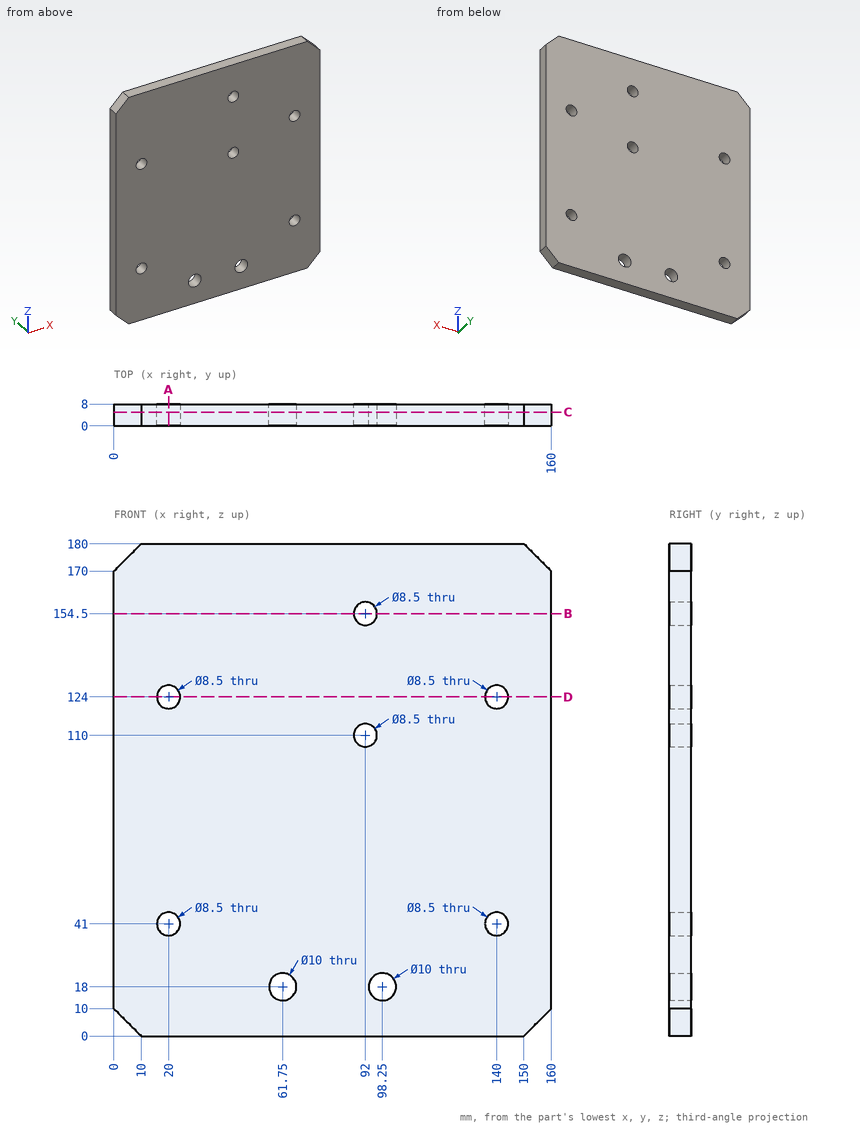
Geometry check sheet. Reference: drawing and pictorial views, mm from the part's lowest x, y, z. Give positions to 0.01 mm unless a question says otherwise; leave off trailing zeros. Order: outer loops, then holes, each group sorted by start corner. A loop starts at its lowest first (then second) coordinate and runs counter-clockwise, first axis right, second up.
1. Section check B-B, the plane z = 154.5. Enter the section's corners in (x, y).
2. Section check D-D, the plane z = 124. Enter the section's corners in (x, y).
3. Section check C-C, the plane y = 5. Give the number of separate pieces and of enclosed holes in the cut face, and give its area (3 significant figures).
4. Section check A-A, the plane x = 20. Enter the section's corners in (y, z).
5. Thickness scan on L1, parallel to Z at x = 92, y = 2; L2, parallel to Z at x = 140, y = 5.75; L3, parallel to Z at x = 61.75, y = 6.5. Record the ranges inside material, lowest first.
Values follow:
1. outline: (0, 0) - (87.75, 0) - (87.75, 8) - (0, 8) - close; (96.25, 0) - (160, 0) - (160, 8) - (96.25, 8) - close
2. outline: (0, 0) - (15.75, 0) - (15.75, 8) - (0, 8) - close; (24.25, 0) - (135.75, 0) - (135.75, 8) - (24.25, 8) - close; (144.25, 0) - (160, 0) - (160, 8) - (144.25, 8) - close
3. separate pieces: 1
3. enclosed holes: 8
3. area: 28,100 mm2
4. outline: (0, 0) - (8, 0) - (8, 36.75) - (0, 36.75) - close; (0, 45.25) - (8, 45.25) - (8, 119.75) - (0, 119.75) - close; (0, 128.25) - (8, 128.25) - (8, 180) - (0, 180) - close
5. L1: z = 0 to 105.75, 114.25 to 150.25, 158.75 to 180
5. L2: z = 0 to 36.75, 45.25 to 119.75, 128.25 to 180
5. L3: z = 0 to 13, 23 to 180
